```python
from build123d import *

# Parameters (mm, degrees)
SKETCH1_W           = 40
SKETCH1_H           = 8
BOSS_EXTRUDE1_DEPTH = 1
SKETCH2_W           = 6
SKETCH2_H           = 0.7
BOSS_EXTRUDE2_DEPTH = 3
SKETCH3_W           = 40
SKETCH3_H           = 0.7
BOSS_EXTRUDE3_DEPTH = 3
CUT_EXTRUDE2_DEPTH  = 3
SKETCH5_R           = 1.5
CUT_EXTRUDE3_DEPTH  = 3
FILLET1_R           = 1


with BuildPart() as part:
    # Sketch1 → Boss-Extrude1 (new body)
    with BuildSketch(Plane.XY):
        Rectangle(SKETCH1_W, SKETCH1_H)
    extrude(amount=BOSS_EXTRUDE1_DEPTH)

    # Sketch2 → Boss-Extrude2 (add)
    with BuildSketch(Plane.XY.offset(1)):
        with Locations((-17, -3.65)):
            Rectangle(SKETCH2_W, SKETCH2_H)
        with Locations((17, -3.65)):
            Rectangle(SKETCH2_W, SKETCH2_H)
    extrude(amount=BOSS_EXTRUDE2_DEPTH)

    # Sketch3 → Boss-Extrude3 (add)
    with BuildSketch(Plane.XY.offset(1)):
        with Locations((0, 3.65)):
            Rectangle(SKETCH3_W, SKETCH3_H)
    extrude(amount=BOSS_EXTRUDE3_DEPTH)

    # Sketch4 → Cut-Extrude2 (cut)
    with BuildSketch(Plane.XY.offset(1)):
        Polygon((-12, 1), (12, 1), (14, -3.3), (14, -4), (-14, -4), (-14, -3.3), align=None)
    extrude(amount=-CUT_EXTRUDE2_DEPTH, mode=Mode.SUBTRACT)

    # Sketch5 → Cut-Extrude3 (cut)
    with BuildSketch(Plane.XY.offset(1)):
        with Locations((16, 0)):
            Circle(SKETCH5_R)
        with Locations((-16, 0)):
            Circle(SKETCH5_R)
    extrude(amount=-CUT_EXTRUDE3_DEPTH, mode=Mode.SUBTRACT)

    # Fillet1
    fillet1_edges = [part.edges().sort_by_distance(p)[0] for p in [
        (-14, -3.65, 4),
        (-20, -3.65, 4),
        (14, -3.65, 4),
        (20, -3.65, 4),
        (20, 3.65, 4),
        (-20, 3.65, 4),
        (17, -4, 0),
        (-17, -4, 0),
        (0, 4, 0),
    ]]
    fillet(fillet1_edges, radius=FILLET1_R)


solid = part.part
```
Model file for the job. Use its own axes, mm. A direction names the side the tool comes from. Give positions to 0.01 mm unless a question says otherwise; leave off trailing zeros. Order: outer loops, then holes, each group sorted by start corner. A loop starts at its lowest first (then second) coordinate and runs counter-clockwise, first axis right, second up.
1) Saw through at B-B, the plane z = 2.35. Write the cut outline in (x, y), then the cut area to 3 significant figures.
2) Mould opens along Y. For faces 4 (the flat face through (-17, -4, 2)), 5 (the flat face through (17, -3.3, 2)), 6 (the flat face through (-0.3, 1.4, 0)) say: +Y half, -Y half, draft (parallel to the pull), parting line (faces both ways), or undercut.
3) 3-axis set-ups, long thin cutter, end or side, ignore diameter. For faces 1 (the flat face through (-13.014, -1.18, 0.507)), 2 (the cylindrical face through (-14.301, -3.645, 3.715)), 3 (the flat face through (-17, -3.3, 2)): which of +Z, -Z, +X, -X, +Y, -Y reach the whole face in a straight line?
4) Saw through at D-D, the plane x = -13. Write the cut outline in (y, z).
5) Saw through at C-C, the plane y = 0.5. Write the cut outline in (x, z), then the cut area to 3 significant figures.
6) Wall check: probe 1 along Y at (x, z) = (-15, 1.05); probe 2 along Y at (x, z) = (1.5, 1.5); probe 3 along X at (y, z) = (-0.75, 0.65). Give the ranges that are in metal, low to high.
7) Pin check, flat tips, straight feed: pin 1 (0.9 mm diameter, centred on x = 2.5, z = 3, fed in from -Y); pin 2 (1 mm diameter, centred on x = -7, y = 2.5, fed in from +Z). Stop position of each tip, or through.
8) Saw through at A-A, the plane x = 16. Write the cut outline in (y, z), then the cut area to 3 significant figures.
Computed:
1. outline: (-20, -4) - (-14, -4) - (-14, -3.3) - (-20, -3.3) - close; (-20, 3.3) - (20, 3.3) - (20, 4) - (-20, 4) - close; (14, -4) - (20, -4) - (20, -3.3) - (14, -3.3) - close
1. area: 36.4 mm2
2. face 4: -Y half
2. face 5: undercut
2. face 6: draft
3. face 1: +Z, -Z, -Y
3. face 2: +Z, -Y
3. face 3: +Z, +X, -X
4. outline: (-1.15, 0) - (3, 0) arc R1 ccw to (4, 1) - (4, 4) - (3.3, 4) - (3.3, 1) - (-1.15, 1) - close
5. outline: (-20, 0) - (-17.41, 0) - (-17.41, 1) - (-20, 1) - close; (-14.59, 0) - (-12.23, 0) - (-12.23, 1) - (-14.59, 1) - close; (12.23, 0) - (14.59, 0) - (14.59, 1) - (12.23, 1) - close; (17.41, 0) - (20, 0) - (20, 1) - (17.41, 1) - close
5. area: 9.88 mm2
6. probe 1: y = -4 to -3.3, 3.3 to 4
6. probe 2: y = 3.3 to 4
6. probe 3: x = -20 to -17.3, -14.7 to -12.81, 12.81 to 14.7, 17.3 to 20
7. pin 1: stops at y = 3.3
7. pin 2: stops at z = 1
8. outline: (-4, 1) arc R1 ccw to (-3, 0) - (-1.5, 0) - (-1.5, 1) - (-3.3, 1) - (-3.3, 4) - (-4, 4) - close; (1.5, 0) - (3, 0) arc R1 ccw to (4, 1) - (4, 4) - (3.3, 4) - (3.3, 1) - (1.5, 1) - close
8. area: 8.77 mm2
